from build123d import *

# Parameters (mm, degrees)
SKETCH1_W               = 8
SKETCH1_H               = 8
BOSS_EXTRUDE1_DEPTH     = 3
CUT_EXTRUDE1_DEPTH      = 12.704699911
CUT_EXTRUDE1_DEPTH_BACK = 12.704699911
CUT_EXTRUDE2_DEPTH      = 11
SKETCH4_R               = 1.8
CUT_EXTRUDE3_DEPTH      = 0.8
SKETCH5_W               = 8
SKETCH5_H               = 1
BOSS_EXTRUDE2_DEPTH     = 2
FILLET1_R               = 4
CUT_EXTRUDE4_DEPTH      = 0.4
CUT_EXTRUDE5_DEPTH      = 0.4


with BuildPart() as part:
    # Sketch1 → Boss-Extrude1 (new body)
    with BuildSketch(Plane(origin=(0, 0, 0), x_dir=(1, 0, 0), z_dir=(0, 1, 0))):
        with Locations((4, 4)):
            Rectangle(SKETCH1_W, SKETCH1_H)
    extrude(amount=BOSS_EXTRUDE1_DEPTH)

    # Sketch2 → Cut-Extrude1 (cut, two sides: drawn at the far end of the back side and taken through both)
    with BuildSketch(Plane.XY.offset(-CUT_EXTRUDE1_DEPTH_BACK)):
        Polygon((0, 0), (0.6, 3), (0, 3), align=None)
        Polygon((8, 0), (7.4, 3), (8, 3), align=None)
    extrude(amount=CUT_EXTRUDE1_DEPTH + CUT_EXTRUDE1_DEPTH_BACK, mode=Mode.SUBTRACT)

    # Sketch3 → Cut-Extrude2 (cut)
    with BuildSketch(Plane(origin=(0, 0, 0), x_dir=(0, 0, -1), z_dir=(1, 0, 0))):
        Polygon((0, 0), (0.6, 3), (0, 3), align=None)
        Polygon((8, 3), (7.4, 3), (8, 0), align=None)
    extrude(amount=CUT_EXTRUDE2_DEPTH, mode=Mode.SUBTRACT)

    # Sketch4 → Cut-Extrude3 (cut)
    with BuildSketch(Plane.XZ):
        with Locations(Location((4, -3.75, 0), (0, 0, 270))):
            Circle(SKETCH4_R)
    extrude(amount=-CUT_EXTRUDE3_DEPTH, mode=Mode.SUBTRACT)

    # Sketch5 → Boss-Extrude2 (add)
    with BuildSketch(Plane.XZ):
        with Locations((4, -7.5)):
            Rectangle(SKETCH5_W, SKETCH5_H)
    extrude(amount=BOSS_EXTRUDE2_DEPTH)

    # Fillet1
    # the kernel refuses this fillet: 4 mm, written as the material it takes off along each edge
    with BuildSketch(Plane(origin=(8, -2, -16.660254038), x_dir=(0, 1, 0), z_dir=(0, 0, 1)), Plane(origin=(0, -2, 1.660254038), x_dir=(0, 1, 0), z_dir=(0, 0, -1))) as fillet1_piece_1:
        with BuildLine():
            CenterArc((4, 3.464101615), FILLET1_R, 180, 60)
            Line((0, 3.464101615), (-0.08, 3.464101615))
            Line((-0.08, 3.464101615), (-0.08, 0))
            Line((-0.08, 0), (0, -0.08))
            ThreePointArc((0, -0.08), (1, -0.08), (1.96, -0.069282032))
            Line((1.96, -0.069282032), (2, 0))
        make_face()
    extrude(amount=18.320508076, mode=Mode.SUBTRACT)

    # Sketch6 → Cut-Extrude4 (cut)
    with BuildSketch(Plane(origin=(0, 3, 0), x_dir=(1, 0, 0), z_dir=(0, 1, 0))):
        with BuildLine():
            Line((2.413140262, 5.995145478), (3.182371031, 5.995145478))
            Line((3.182371031, 5.995145478), (3.182371031, 3.824472401))
            add(Edge.make_bspline(
                [(3.182371031, 3.824472401), (3.182664695, 3.783339968), (3.183225327, 3.704814249), (3.183611242, 3.59262518), (3.18574694, 3.491896749), (3.190378411, 3.402466647), (3.193557117, 3.32438048), (3.199459629, 3.257623918), (3.205347836, 3.202222959), (3.211072588, 3.16927001), (3.213621031, 3.154600607)],
                knots=[0, 0, 0, 0, 1.470600056, 2.807515117, 4.011048972, 5.072079398, 6.00911328, 6.804506435, 7.467811572, 8, 8, 8, 8], degree=3))
            add(Edge.make_bspline(
                [(3.213621031, 3.154600607), (3.224127628, 3.115054038), (3.244816443, 3.03718185), (3.301842427, 2.930732637), (3.377172946, 2.83690436), (3.454012852, 2.769989694), (3.523520467, 2.722632459), (3.582561491, 2.693810163), (3.645203631, 2.667536787), (3.712771176, 2.647377448), (3.784538951, 2.629737301), (3.861373833, 2.619537644), (3.942627383, 2.611709661), (3.998321517, 2.610930314), (4.026922313, 2.610530094)],
                knots=[0, 0, 0, 0, 1.376921055, 2.711331395, 4.038631339, 5.418057255, 6.132954575, 6.870556231, 7.630397752, 8.422890386, 9.247036838, 10.121396817, 11.035274583, 12, 12, 12, 12], degree=3))
            add(Edge.make_bspline(
                [(4.026922313, 2.610530094), (4.055777389, 2.611053435), (4.111957634, 2.612072369), (4.193372399, 2.618140476), (4.269330983, 2.629588903), (4.339786919, 2.644600001), (4.40511233, 2.663571514), (4.464786061, 2.687591678), (4.518714075, 2.716497769), (4.582078678, 2.760066391), (4.650258908, 2.821527538), (4.715873674, 2.905091818), (4.762833649, 2.997337694), (4.784859868, 3.081565077), (4.796180605, 3.154949811), (4.803077806, 3.219164001), (4.809385646, 3.291832182), (4.815113647, 3.372755319), (4.819030865, 3.461994153), (4.821149619, 3.559774375), (4.82281709, 3.666080391), (4.823198873, 3.739802878), (4.823396672, 3.777998042)],
                knots=[0, 0, 0, 0, 1.036876239, 2.018776863, 2.930845756, 3.794842666, 4.605604932, 5.371924355, 6.101864688, 6.799283669, 8.1310906, 9.382718023, 10.597336334, 11.822035891, 12.492591141, 13.265194674, 14.141890321, 15.11351293, 16.179860579, 17.351049011, 18.627594861, 20, 20, 20, 20], degree=3))
            Line((4.823396672, 3.777998042), (4.823396672, 5.995145478))
            Line((4.823396672, 5.995145478), (5.592627441, 5.995145478))
            Line((5.592627441, 5.995145478), (5.592627441, 3.902998042))
            add(Edge.make_bspline(
                [(5.592627441, 3.902998042), (5.592528847, 3.845305157), (5.592339402, 3.734449864), (5.589381475, 3.574956755), (5.583094941, 3.428628514), (5.577830511, 3.295214312), (5.567675642, 3.175054503), (5.557043529, 3.068074376), (5.543346947, 2.974292627), (5.523815493, 2.867696041), (5.490991615, 2.748101531), (5.438090809, 2.615994056), (5.370481989, 2.495804532), (5.288434562, 2.387071806), (5.192421188, 2.289363714), (5.081004269, 2.203064381), (4.955329501, 2.127124651), (4.84016309, 2.072443299), (4.739752735, 2.035622669), (4.65797018, 2.010704116), (4.570444093, 1.989952175), (4.477277128, 1.973483664), (4.378429252, 1.959598273), (4.273864574, 1.950325107), (4.163741291, 1.944537997), (4.088628699, 1.944091898), (4.050159493, 1.943863427)],
                knots=[0, 0, 0, 0, 1.415574045, 2.719986624, 3.913607924, 5.00929969, 5.995467356, 6.871900228, 7.64671288, 8.320227872, 9.530145585, 10.682614022, 11.803571353, 12.90325401, 14.015460715, 15.154679255, 16.351678057, 17.612271512, 18.275764165, 18.974412946, 19.708786676, 20.481351116, 21.295095879, 22.157200529, 23.056203067, 24, 24, 24, 24], degree=3))
            add(Edge.make_bspline(
                [(4.050159493, 1.943863427), (4.00394899, 1.944454117), (3.914432357, 1.945598373), (3.784491522, 1.950702797), (3.663419731, 1.961238523), (3.550836598, 1.975478544), (3.446788608, 1.993784557), (3.351012543, 2.015669281), (3.264273035, 2.043328483), (3.160959321, 2.082832512), (3.045798952, 2.143260432), (2.920442018, 2.223870786), (2.810400187, 2.314853884), (2.716640343, 2.415320705), (2.638260762, 2.521740618), (2.574552012, 2.631810814), (2.523497916, 2.743696672), (2.502164616, 2.821459533), (2.491665903, 2.859728812)],
                knots=[0, 0, 0, 0, 1.128613534, 2.186292659, 3.174878439, 4.095586888, 4.95671962, 5.754129884, 6.492676435, 7.178284149, 8.453103036, 9.659838108, 10.813193309, 11.929983019, 13.007587775, 14.033493319, 15.032227051, 16, 16, 16, 16], degree=3))
            add(Edge.make_bspline(
                [(2.491665903, 2.859728812), (2.48524032, 2.889857793), (2.471705989, 2.953319061), (2.456334745, 3.054210037), (2.442311642, 3.165307899), (2.432733679, 3.286744058), (2.423654648, 3.418133217), (2.417136225, 3.559723113), (2.414455843, 3.711481594), (2.413587623, 3.816192051), (2.413140262, 3.870145478)],
                knots=[0, 0, 0, 0, 0.728071598, 1.533551606, 2.411422299, 3.374601532, 4.412367648, 5.524718474, 6.72457895, 8, 8, 8, 8], degree=3))
            Line((2.413140262, 3.870145478), (2.413140262, 5.995145478))
        make_face()
    extrude(amount=-CUT_EXTRUDE4_DEPTH, mode=Mode.SUBTRACT)

    # Sketch7 → Cut-Extrude5 (cut)
    with BuildSketch(Plane(origin=(0, 3, 0), x_dir=(1, 0, 0), z_dir=(0, 1, 0))):
        with BuildLine():
            Line((5.850386773, 2.400368579), (5.850386773, 2.746522425))
            Line((5.850386773, 2.746522425), (7.02730985, 2.746522425))
            Line((7.02730985, 2.746522425), (7.02730985, 2.492676271))
            add(Edge.make_bspline(
                [(7.02730985, 2.492676271), (7.015032321, 2.480184286), (6.989793248, 2.454504354), (6.953640746, 2.41247659), (6.916952595, 2.366869092), (6.880495981, 2.317067299), (6.84313767, 2.263857918), (6.806519427, 2.206220957), (6.769380335, 2.144904141), (6.719379376, 2.058171383), (6.660934493, 1.944871602), (6.599102899, 1.804034186), (6.546425212, 1.658871525), (6.510353845, 1.535182236), (6.485981829, 1.436045461), (6.470058334, 1.363554301), (6.45665413, 1.293103137), (6.44574982, 1.224568153), (6.437611625, 1.157918082), (6.431181064, 1.093384645), (6.428008496, 1.030810475), (6.427540351, 0.989794441), (6.42730985, 0.969599348)],
                knots=[0, 0, 0, 0, 0.628545797, 1.29210959, 1.98878689, 2.729126096, 3.507039704, 4.322017351, 5.179550397, 6.080149501, 7.915136253, 9.752312618, 11.597470118, 13.454141581, 14.373891568, 15.261584755, 16.117868869, 16.947726723, 17.752002974, 18.527724242, 19.275094557, 20, 20, 20, 20], degree=3))
            Line((6.42730985, 0.969599348), (6.081156004, 0.969599348))
            add(Edge.make_bspline(
                [(6.081156004, 0.969599348), (6.082313464, 1.000264514), (6.084641243, 1.061935513), (6.093350513, 1.15450167), (6.107029358, 1.247412503), (6.124019401, 1.340882746), (6.146450494, 1.434684851), (6.172051243, 1.529166286), (6.203062702, 1.623822431), (6.237825714, 1.718472296), (6.276202253, 1.812217257), (6.31802728, 1.903894573), (6.363192674, 1.992932291), (6.411111069, 2.079643245), (6.462339924, 2.16374848), (6.516917811, 2.245156666), (6.574070556, 2.324456683), (6.614935451, 2.375068877), (6.635362734, 2.400368579)],
                knots=[0, 0, 0, 0, 0.943249748, 1.896978291, 2.856365892, 3.829648507, 4.816416106, 5.820376826, 6.838120354, 7.877341886, 8.919613352, 9.951365796, 10.974227495, 11.988073359, 12.996274698, 14.000568529, 15.000536908, 16, 16, 16, 16], degree=3))
            Line((6.635362734, 2.400368579), (5.850386773, 2.400368579))
        make_face()
    extrude(amount=-CUT_EXTRUDE5_DEPTH, mode=Mode.SUBTRACT)


solid = part.part
Part model, mm, in its own coordinate system. A direction names the side the tool comes from. Round coordinates to 2 decimals unless told otherwise and drop trailing zeros. Order: outer loops, then holes, each group sorted by start corner. A loop starts at its lowest first (then second) coordinate and runs counter-clockwise, first axis right, second up. Notation, with made-up numbers: (-26.5, 41.5) -> (-3.5, 41.5) arc R27 ccw to (-3.5, 60.5) -> close; hole circle Ø2 at (57, 89). An arc over 180 degrees is marked (long way). Put each result on its own line as item: value.
Q1. Wall check: line 1 (Y direction, x = 3.75, z = -1.5); line 2 (Z direction, x = 3.5, y = -1.2); line 3 (Y direction, x = 2.75, z = -5). Give the ranges that are in metal, low to high. Write a range as [from, to].
From the geometry:
line 1: y = [0, 3]
line 2: z = [-8, -7]
line 3: y = [0.8, 2.6]
Q2. Band-saw the part on B-B (y = 2.45). Give the cut face in (x, z), and give its area (3 significant figures).
From the geometry:
outline: (0.49, -7.51) -> (7.51, -7.51) -> (7.51, -0.49) -> (0.49, -0.49) -> close
area: 49.3 mm2
Q3. Pull direction X, two halves, no side cores. Call faces 5 (the face through (6.51, -1.48, -7.51)), 6 (the face through (4, -2, -7.5)), 7 (the face through (4.541, 0.394, -5.467)): pulls with the +X half, pulls with the -X half, needs draft (parallel to the pull), parting line crosses it, or undercut.
From the geometry:
face 5: pulls with the +X half
face 6: needs draft
face 7: undercut
Q4. Band-saw the part on C-C (y = -0.85). Give the cut face in (x, z).
From the geometry:
outline: (0.66, -8) -> (7.34, -8) -> (7.34, -7) -> (0.66, -7) -> close
Q5. Pin check, flat tips, straight feed: pin 1 Ø3 at (x, z) = (4.5, -3.5) entering from -Y; pin 2 Ø1 at (y, z) = (1.5, -2.5) entering from +X; pin 3 Ø1 at (y, z) = (-1, -7) entering from -X. Stop position of each tip, or through.
From the geometry:
pin 1: stops at y = 0
pin 2: stops at x = 7.8
pin 3: stops at x = 0.34
Q6. Band-saw the part on A-A (y = 0.6). Give the cut face in (x, z), and give its area (3 significant figures).
From the geometry:
outline: (0.12, -7.88) -> (7.88, -7.88) -> (7.88, -0.12) -> (0.12, -0.12) -> close; hole circle Ø3.6 at (4, -3.75)
area: 50.0 mm2
Q7. Tool access for faces 1 (the face through (4, 0.8, -4)), 2 (the face through (1.49, -1.48, -7.49)), 3 (the face through (3, 2.6, -4)), 4 (the face through (4, -1, -7)): list every direction of +Z, -Z, +X, -X, +Y, -Y with a clear straight run to the whole face (end or side of a thin tool).
From the geometry:
face 1: -Y
face 2: +Z, -Z, -X, -Y
face 3: +Y
face 4: +Z, +X, -X, -Y
